```python
from build123d import *

# Parameters (mm, degrees)
SKETCH1_W           = 24
SKETCH1_H           = 10
BOSS_EXTRUDE1_DEPTH = 1
SKETCH2_W           = 3
SKETCH2_H           = 6.1
BOSS_EXTRUDE2_DEPTH = 3.25
SKETCH3_R           = 3.25
CUT_EXTRUDE1_DEPTH  = 3
FILLET1_R           = 0.2
SKETCH4_W           = 1
SKETCH4_H           = 6.1
BOSS_EXTRUDE3_DEPTH = 1


with BuildPart() as part:
    # Sketch1 → Boss-Extrude1 (new body)
    with BuildSketch(Plane(origin=(0, 0, 0), x_dir=(1, 0, 0), z_dir=(0, 1, 0))):
        with Locations((-12, 5)):
            Rectangle(SKETCH1_W, SKETCH1_H)
    extrude(amount=BOSS_EXTRUDE1_DEPTH)

    # Sketch2 → Boss-Extrude2 (add)
    with BuildSketch(Plane(origin=(0, 1, 0), x_dir=(1, 0, 0), z_dir=(0, 1, 0))):
        with Locations((-0.5, 5.6)):
            Rectangle(SKETCH2_W, SKETCH2_H)
    extrude(amount=BOSS_EXTRUDE2_DEPTH)

    # Sketch3 → Cut-Extrude1 (cut)
    with BuildSketch(Plane(origin=(-2, 0, 0), x_dir=(0, 0, -1), z_dir=(1, 0, 0))):
        with Locations((5.5, 5)):
            Circle(SKETCH3_R)
    extrude(amount=CUT_EXTRUDE1_DEPTH, mode=Mode.SUBTRACT)

    # Fillet1
    fillet1_edges = [part.edges().sort_by_distance(p)[0] for p in [
        (-0.5, 3.63618183, -2.55),
        (-0.5, 4.2, -8.65),
    ]]
    fillet(fillet1_edges, radius=FILLET1_R)

    # Sketch4 → Boss-Extrude3 (add)
    with BuildSketch(Plane.XZ.offset(-1)):
        with Locations((0.5, -5.6)):
            Rectangle(SKETCH4_W, SKETCH4_H)
    extrude(amount=BOSS_EXTRUDE3_DEPTH)


solid = part.part
```
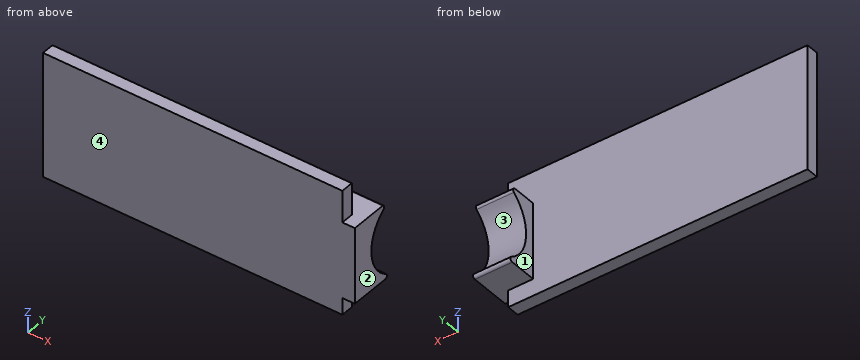
Could you check a few things on this model? Use its own coordinates, in mm. Face numbers are marked on the shaded views. A direction names the side the tool comes from. Coordinates: 2 decimals unless noted, no trailing zeros. Loops run counter-clockwise (first coordinate to the right, second up) from the corner with the lowest first, then second, coordinate; pieces in that order, holes last.
1) Thinking about a two-plate mould opening in Z: for the marked faces 3 and 4, which applies, released by +Z, released by -Z, zero draft, split by the parting line, or undercut?
Reported:
face 3: undercut
face 4: zero draft
2) Imagine slicing it at D-D (x = -9.75). List the corners of the cut face in (y, z) for me, and give its area (3 significant figures).
Reported:
outline: (0, -10) - (1, -10) - (1, 0) - (0, 0) - close
area: 10.0 mm2
3) Which directions (+Z, -Z, +X, -X, +Y, -Y) give clear straight access to the entire face, cutting with the end or side of a thin tool? Please do the marked faces 1 and 2.
Reported:
face 1: +Z, -Z, -X, +Y
face 2: +Z, -Z, +X, +Y, -Y
4) Imagine slicing it at A-A (y = 2.6). List the corners of the cut face in (x, z) for me, and give its area (3 significant figures).
Reported:
outline: (-2, -8.65) - (1, -8.65) - (1, -7.69) - (-2, -7.69) - close; (-2, -3.31) - (1, -3.31) - (1, -2.55) - (-2, -2.55) - close
area: 5.15 mm2
5) Imagine slicing it at C-C (z = -6.75). List the corners of the cut face in (x, y) for me, and give its area (3 significant figures).
Reported:
outline: (-24, 0) - (1, 0) - (1, 2) - (-2, 2) - (-2, 1) - (-24, 1) - close
area: 28.0 mm2
6) Imagine slicing it at B-B (y = 0.45). List the corners of the cut face in (x, z) for me, and give its area (3 significant figures).
Reported:
outline: (-24, -10) - (0, -10) - (0, -8.65) - (1, -8.65) - (1, -2.55) - (0, -2.55) - (0, 0) - (-24, 0) - close
area: 246 mm2
7) Please list where these lines run through material, in increasing order: line 1 along Y through (x, z) = (-7, -8.5); line 2 along X through (y, z) = (1.85, -7.5).
Reported:
line 1: y = 0 to 1
line 2: x = -2 to 1
8) Will these pins go through, and if not, where does the flat tip stop? pin 1 Ø2 at (x, z) = (-14.5, -4) entering from +Y; pin 2 Ø0.8 at (y, z) = (0.5, -2) entering from +X; pin 3 Ø1.9 at (y, z) = (2, -6.5) entering from -X.
Reported:
pin 1: stops at y = 1
pin 2: stops at x = 0
pin 3: stops at x = -2
